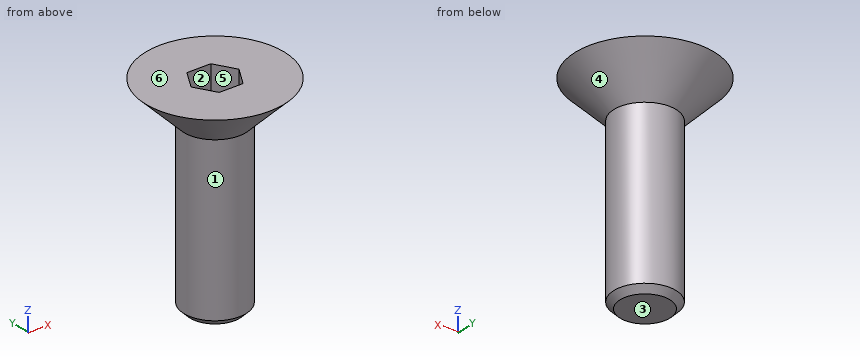
from build123d import *

# Parameters (mm, degrees)
CUT_EXTRUDE_1_DEPTH = 2
CHAMFER_1_SIZE      = 0.3


with BuildPart() as part:
    # Эскиз1 → Повернуть1 (revolve)
    with BuildSketch(Plane(origin=(0, 0, 0), x_dir=(0, 0, -1), z_dir=(1, 0, 0))):
        Polygon((0, 0), (0, 3.36), (1.86, 1.5), (10, 1.5), (10, 0), align=None)
    revolve(axis=Axis((0, 0, -10), (0, 0, 1)))

    # Эскиз2 → Вырез-Вытянуть1 (cut)
    with BuildSketch(Plane.XY):
        Polygon((1.154700538, 0), (0.577350269, 1), (-0.577350269, 1), (-1.154700538, 0), (-0.577350269, -1), (0.577350269, -1), align=None)
    extrude(amount=-CUT_EXTRUDE_1_DEPTH, mode=Mode.SUBTRACT)

    # Фаска1
    chamfer_1_edges = [part.edges().sort_by_distance(p)[0] for p in [
        (0, -1.5, -10),
    ]]
    chamfer(chamfer_1_edges, length=CHAMFER_1_SIZE)


solid = part.part
Part model, mm, in its own coordinate system. Face numbers are marked on the shaded views. A direction names the side the tool comes from. Coordinates: 2 decimals unless noted, no trailing zeros. Loops run counter-clockwise (first coordinate to the right, second up) from the corner with the lowest first, then second, coordinate; pieces in that order, holes last. Notation, with made-up numbers: M -20.5,69 L -2.5,69 A9 ccw -2.5,81 Z; hole C -27,33 d8. An arc over 180 degrees is marked long. Use a Markdown table: item, result. Add a question column.
Q1. Cut at A-A (z = -0.25). Write the cut outline in (x, y), and give its area (3 significant figures).
Q2. Pin check, flat tips, straight feed: P1, Ø3, axis at x = -1.5, z = -6.5, coming from the +Y side; P2, Ø0.9, axis at x = 0.5, z = -1, coming from the +Y side; P3, Ø2, axis at x = 1.5, z = -3, coming from the +Y side. Stop position of each tip, or through.
Q3. Which spindle directions (+Z, -Z, +X, -X, +Y, -Y) get a long thin tool onto all of the face, cutting with end or side? Do the marked faces 1, 2 and 3. Say none if no direction does.
Q4. Mould opens along X. For the marked faces 4, 5 and 6 say: +X half, -X half, draft (parallel to the pull), parting line (faces both ways), or undercut.
Q5. Cut at C-C (z = -7). Write the cut outline in (x, y), and give its area (3 significant figures).
Q6. Cut at B-B (x = 0). Write the cut outline in (y, z).
Q7. Probe L1, parallel to Z at x = 0, y = 0; L2, parallel to X at y = 0, z = -8.25; L3, parallel to Y at x = -0.25, z = -0.25. List the from-to ranges inside material, lowest first.
Worked out:
| question | item | result |
|---|---|---|
| 1 | outline | C 0,0 d6.22; hole M -1.15,0 L -0.58,-1 L 0.58,-1 L 1.15,0 L 0.58,1 L -0.58,1 Z |
| 1 | area | 26.9 mm2 |
| 2 | P1 | stops at y = 1.5 |
| 2 | P2 | stops at y = 2.77 |
| 2 | P3 | stops at y = 1.41 |
| 3 | face 1 | -Z |
| 3 | face 2 | +Z |
| 3 | face 3 | -Z, +X, -X, +Y, -Y |
| 4 | face 4 | parting line |
| 4 | face 5 | undercut |
| 4 | face 6 | draft |
| 5 | outline | C 0,0 d3 |
| 5 | area | 7.07 mm2 |
| 6 | outline | M -3.36,0 L -1.5,-1.86 L -1.5,-9.7 L -1.2,-10 L 1.2,-10 L 1.5,-9.7 L 1.5,-1.86 L 3.36,0 L 1,0 L 1,-2 L -1,-2 L -1,0 Z |
| 7 | L1 | z = -10 to -2 |
| 7 | L2 | x = -1.5 to 1.5 |
| 7 | L3 | y = -3.1 to -1, 1 to 3.1 |
